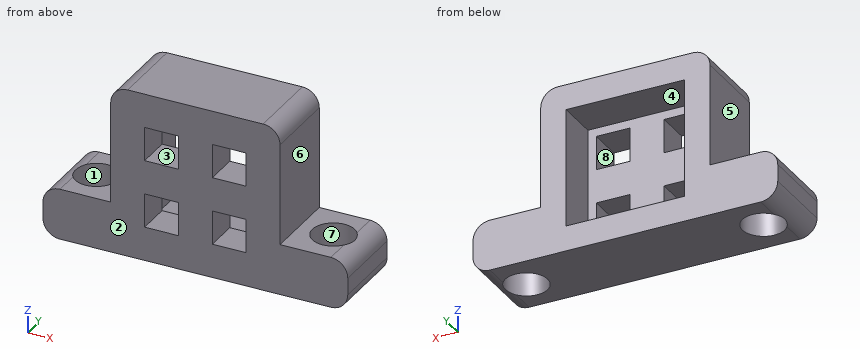
```python
from build123d import *

# Parameters (mm, degrees)
ESBO_O1_W                = 10
ESBO_O1_H                = 10
ESBO_O1_W_2              = 2
ESBO_O1_H_2              = 2
RESSALTO_EXTRUS_O1_DEPTH = 2
ESBO_O2_W                = 10
ESBO_O2_H                = 10
RESSALTO_EXTRUS_O2_DEPTH = 2.5
ESBO_O3_W                = 4
ESBO_O3_H                = 4.5
ESBO_O3_R                = 1.25
RESSALTO_EXTRUS_O3_DEPTH = 3
FILETE1_R                = 1


with BuildPart() as part:
    # Esboço1 → Ressalto-extrusão1 (new body)
    with BuildSketch(Plane(origin=(0, 0, 0), x_dir=(1, 0, 0), z_dir=(0, 1, 0))):
        Rectangle(ESBO_O1_W, ESBO_O1_H)
        with Locations((2, 2)):
            Rectangle(ESBO_O1_W_2, ESBO_O1_H_2, mode=Mode.SUBTRACT)
        with Locations((-2, 2)):
            Rectangle(ESBO_O1_W_2, ESBO_O1_H_2, mode=Mode.SUBTRACT)
        with Locations((2, -2)):
            Rectangle(ESBO_O1_W_2, ESBO_O1_H_2, mode=Mode.SUBTRACT)
        with Locations((-2, -2)):
            Rectangle(ESBO_O1_W_2, ESBO_O1_H_2, mode=Mode.SUBTRACT)
    extrude(amount=RESSALTO_EXTRUS_O1_DEPTH)

    # Esboço2 → Ressalto-extrusão2 (add)
    with BuildSketch(Plane(origin=(0, 2, 0), x_dir=(1, 0, 0), z_dir=(0, 1, 0))):
        Rectangle(ESBO_O2_W, ESBO_O2_H)
        Polygon((-1, -3.5), (3.5, -3.5), (3.5, 3.5), (1, 3.5), (-3.5, 3.5), (-3.5, 1), (-3.5, -3.5), align=None, mode=Mode.SUBTRACT)
    extrude(amount=RESSALTO_EXTRUS_O2_DEPTH)

    # Esboço3 → Ressalto-extrusão3 (add)
    # profile 1 of 2: a face of its own
    with BuildSketch(Plane(origin=(0, 0, -5), x_dir=(-1, 0, 0), z_dir=(0, 0, -1))):
        with Locations((-7, 2.25)):
            Rectangle(ESBO_O3_W, ESBO_O3_H)
        with Locations((-7, 2.25)):
            Circle(ESBO_O3_R, mode=Mode.SUBTRACT)
    # profile 2 of 2: a face of its own
    with BuildSketch(Plane(origin=(0, 0, -5), x_dir=(-1, 0, 0), z_dir=(0, 0, -1))):
        with Locations((7, 2.25)):
            Rectangle(ESBO_O3_W, ESBO_O3_H)
        with Locations((7, 2.25)):
            Circle(ESBO_O3_R, mode=Mode.SUBTRACT)
    extrude(amount=-RESSALTO_EXTRUS_O3_DEPTH)

    # Filete1
    # the kernel refuses this fillet: 1 mm, written as the material it takes off along each edge
    with BuildSketch(Plane(origin=(9, 7, -2), x_dir=(-1, 0, 0), z_dir=(0, -1, 0)), Plane(origin=(-9, 7, -5), x_dir=(1, 0, 0), z_dir=(0, -1, 0)), Plane(origin=(5, 7, 5), x_dir=(-1, 0, 0), z_dir=(0, -1, 0))) as filete1_piece_1:
        with BuildLine():
            CenterArc((FILETE1_R, FILETE1_R), FILETE1_R, 180, 90)
            Line((0, FILETE1_R), (0, 0))
            Line((0, 0), (FILETE1_R, 0))
        make_face()
    extrude(amount=9.5, mode=Mode.SUBTRACT)
    with BuildSketch(Plane(origin=(9, 7, -5), x_dir=(-1, 0, 0), z_dir=(0, -1, 0)), Plane(origin=(-9, 7, -2), x_dir=(1, 0, 0), z_dir=(0, -1, 0)), Plane(origin=(-5, -2.5, 5), x_dir=(0, 0, -1), z_dir=(0, 1, 0))) as filete1_piece_2:
        with BuildLine():
            CenterArc((FILETE1_R, -FILETE1_R), FILETE1_R, 90, 90)
            Line((0, -FILETE1_R), (0, 0))
            Line((0, 0), (FILETE1_R, 0))
        make_face()
    extrude(amount=9.5, mode=Mode.SUBTRACT)


solid = part.part
```
Geometry check sheet. Reference: the model listing, model coordinates, mm. Face numbers are marked on the shaded views. A direction names the side the tool comes from. Coordinates: 2 decimals unless noted, no trailing zeros. Order: outer loops, then holes, each group sorted by start corner. A loop starts at its lowest first (then second) coordinate and runs counter-clockwise, first axis right, second up.
Item 1: Tool access check on the marked faces 4, 5, 6, 7 and 8. Record the directions out of +Z, -Z, +X, -X, +Y, -Y that give a thin tool (end or side, any length) a straight path to the whole face; none if there is none.
Item 2: Scan lines: line 1 along X through (y, z) = (0.85, -1.25); line 2 along X through (y, z) = (2.25, -3.45); line 3 along X through (y, z) = (2.25, -3.65). Record each from-to range of solid material in increasing order.
Item 3: Mould release check, pull along Y, two halves, no side actions. Record for the marked faces 1, 2 and 3: released by +Y, released by -Y, zero draft, split by the parting line, or undercut.
Item 4: Depth check by flat-ended pin: pin 1 (2 mm diameter, centred on y = 1.5, z = -1.5, fed in from -X); pin 2 (2 mm diameter, centred on y = 1, z = 2.5, fed in from +X); pin 3 (1.5 mm diameter, centred on x = -6.5, y = 2, fed in from +Z). Enter the tip coordinate at first touch or a pass-through.
Item 5: Section check C-C (y = 3.2). Enter the section's corners in (x, z), plus the area to 3 significant figures.
Item 6: Section check A-A (x = 6.25). Enter the section's corners in (y, z), plus the area to 3 significant figures.
Item 7: Section check B-B (y = 1.7). Count the separate pieces of the cut face and the enclosed holes in it, plus the area to 3 significant figures.
Check sheet entries:
1. face 4: +Y
1. face 5: +Z, -X, +Y, -Y
1. face 6: +Z, +X, +Y, -Y
1. face 7: +Z, -Z
1. face 8: +Y, -Y
2. line 1: x = -5 to -3, -1 to 1, 3 to 5
2. line 2: x = -9 to -8.25, -5.75 to -3.5, 3.5 to 5.75, 8.25 to 9
2. line 3: x = -9 to -8.25, -5.75 to 5.75, 8.25 to 9
3. face 1: undercut
3. face 2: released by -Y
3. face 3: zero draft
4. pin 1: stops at x = -8.87
4. pin 2: stops at x = 5
4. pin 3: stops at z = -2
5. outline: (-9, -4) arc R1 ccw to (-8, -5) - (-7.81, -5) - (-7.81, -2) - (-8, -2) arc R1 ccw to (-9, -3) - close; (-6.19, -5) - (6.19, -5) - (6.19, -2) - (5, -2) - (5, 4) arc R1 ccw to (4, 5) - (-4, 5) arc R1 ccw to (-5, 4) - (-5, -2) - (-6.19, -2) - close; (7.81, -5) - (8, -5) arc R1 ccw to (9, -4) - (9, -3) arc R1 ccw to (8, -2) - (7.81, -2) - close; hole (-3.5, -3.5) - (3.5, -3.5) - (3.5, 3.5) - (-3.5, 3.5) - close
5. area: 64.0 mm2
6. outline: (0, -5) - (1.25, -5) - (1.25, -2) - (0, -2) - close; (3.25, -5) - (4.5, -5) - (4.5, -2) - (3.25, -2) - close
6. area: 7.50 mm2
7. separate pieces: 3
7. enclosed holes: 4
7. area: 93.2 mm2
